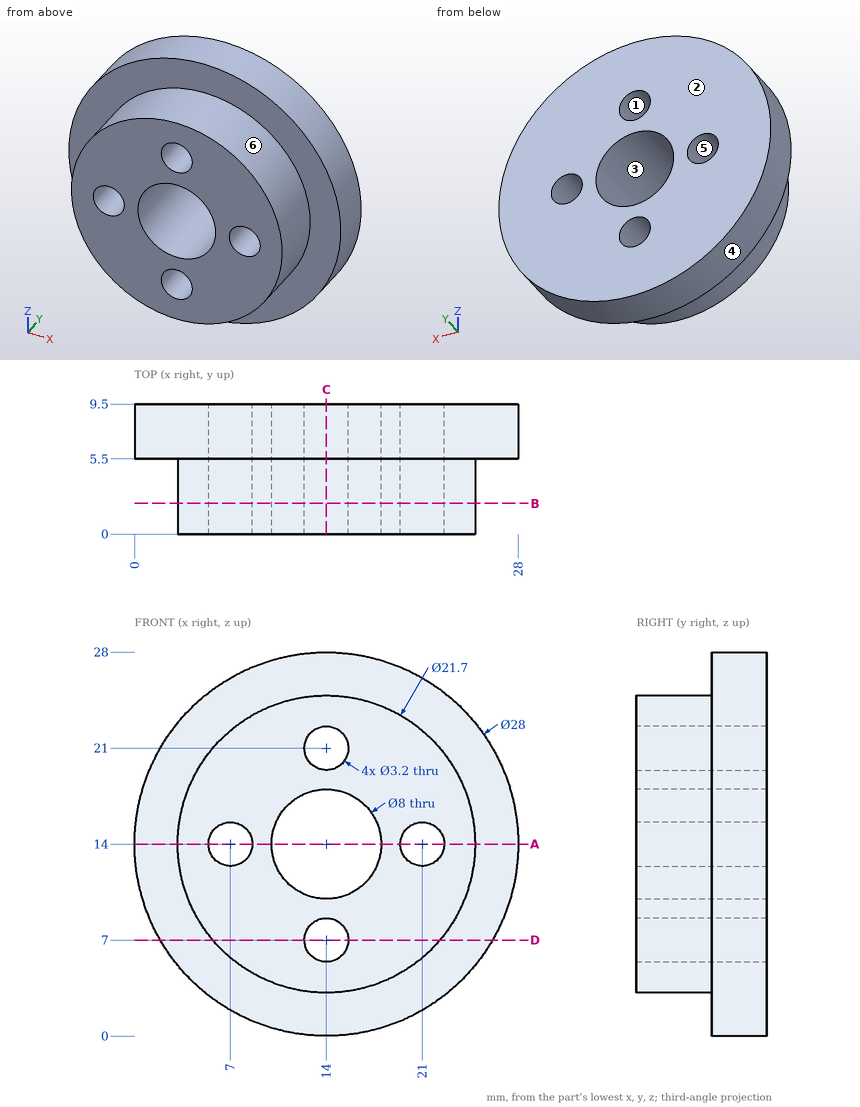
The drawing under review shows one solid part. Ordinate dimensions are in mm from its lowest x, y, z. A direction names the side the tool comes from. Coordinates: 2 decimals unless noted, no trailing zeros. Write each loop counter-clockwise with the first axis right and the second up, starting at its lowest first coordinate (ties: lowest second). Pieces come first, ordered by that corner, then holes. Notation, with made-up numbers: (60.5, 48.25) -> (106.5, 48.25) arc R19 cw to (106.5, 65.25) -> close; hole circle Ø7 at (-39, 40). An arc over 180 degrees is marked (long way). Write each question's results on one line, items separated by ' | '. Start each with the question number.
1) Consider section B-B (y = 2.25). Write out the cut boundary in (x, z).
2) Consider section A-A (z = 14). Write out the cut boundary in (x, y), plus the area to 4 significant figures.
3) Wall thickness on L1, parallel to X at y = 4.5, z = 14; L2, parallel to Z at x = 13.75, y = 3.25; L3, parallel to X at y = 1.25, z = 7.5: over which ranges is each line inside the solid? List them lowest first. Write a range as [from, to].
4) Consider section D-D (z = 7). Write out the cut boundary in (x, y), plus the area to 3 significant figures.
5) The part is to be moulded in two halves that separate along X. For the marked faces 1, 2, 3 and 4, say which applies: +X half, -X half, draft (parallel to the pull), parting line (faces both ways), or undercut.
6) Consider section C-C (x = 14). Write out the cut boundary in (y, z), plus the area to 4 significant figures.
7) Insertion check: pin 1 (2.5 mm diameter, centred on x = 14, z = 7, fed in from -Y); pin 2 (2 mm diameter, centred on x = 21.5, y = 2.5, fed in from +Z). Each pin has a flat end and moves straight along its axis. Give the tip position at first contact, or say it passes through.
8) For the marked faces 5 and 6, list the 3-axis set-ups (+Z, -Z, +X, -X, +Y, -Y) from which the entire face can be reached by the end or side of a thin tool; tool diameter is ignored.
Geometry says:
1) outline: circle Ø21.7 at (14, 14); hole circle Ø3.2 at (7, 14); hole circle Ø8 at (14, 14); hole circle Ø3.2 at (14, 7); hole circle Ø3.2 at (14, 21); hole circle Ø3.2 at (21, 14)
2) outline: (0, 5.5) -> (3.15, 5.5) -> (3.15, 0) -> (5.4, 0) -> (5.4, 9.5) -> (0, 9.5) -> close; (8.6, 0) -> (10, 0) -> (10, 9.5) -> (8.6, 9.5) -> close; (18, 0) -> (19.4, 0) -> (19.4, 9.5) -> (18, 9.5) -> close; (22.6, 0) -> (24.85, 0) -> (24.85, 5.5) -> (28, 5.5) -> (28, 9.5) -> (22.6, 9.5) -> close | area: 94.55 mm^2
3) L1: [3.15, 5.4], [8.6, 10], [18, 19.4], [22.6, 24.85] | L2: [3.15, 5.42], [8.58, 10.01], [17.99, 19.42], [22.58, 24.85] | L3: [5.31, 12.48], [15.52, 22.69]
4) outline: (1.88, 5.5) -> (5.71, 5.5) -> (5.71, 0) -> (12.4, 0) -> (12.4, 9.5) -> (1.88, 9.5) -> close; (15.6, 0) -> (22.29, 0) -> (22.29, 5.5) -> (26.12, 5.5) -> (26.12, 9.5) -> (15.6, 9.5) -> close | area: 158 mm^2
5) face 1: undercut | face 2: draft | face 3: undercut | face 4: parting line
6) outline: (0, 3.15) -> (5.5, 3.15) -> (5.5, 0) -> (9.5, 0) -> (9.5, 5.4) -> (0, 5.4) -> close; (0, 8.6) -> (9.5, 8.6) -> (9.5, 10) -> (0, 10) -> close; (0, 18) -> (9.5, 18) -> (9.5, 19.4) -> (0, 19.4) -> close; (0, 22.6) -> (9.5, 22.6) -> (9.5, 28) -> (5.5, 28) -> (5.5, 24.85) -> (0, 24.85) -> close | area: 94.55 mm^2
7) pin 1: through | pin 2: z = 22.69
8) face 5: +Y, -Y | face 6: -Y
